from build123d import *

# Parameters (mm, degrees)
SKETCH_1_W          = 170
SKETCH_1_H          = 200
SKETCH_1_R          = 1.6
SKETCH_1_W_2        = 65
SKETCH_1_H_2        = 160
EXTRUDE_1_DEPTH     = 5
SKETCH_5_W          = 5
SKETCH_5_H          = 200
EXTRUDE_2_DEPTH     = 20
SKETCH_4_R          = 1.75
CUT_EXTRUDE_1_DEPTH = 30
SKETCH_6_W          = 5
SKETCH_6_H          = 200
EXTRUDE_3_DEPTH     = 20
CUT_EXTRUDE_2_DEPTH = 20


with BuildPart() as part:
    # 草图1 → 凸台-拉伸1 (new body)
    with BuildSketch(Plane.XY):
        with Locations((0.050009972, 0.429149843)):
            Rectangle(SKETCH_1_W, SKETCH_1_H)
        with Locations((-74.949990028, 60.429149843)):
            Circle(SKETCH_1_R, mode=Mode.SUBTRACT)
        with Locations((-74.949990028, -59.570850157)):
            Circle(SKETCH_1_R, mode=Mode.SUBTRACT)
        with Locations((75.050009972, -59.570850157)):
            Circle(SKETCH_1_R, mode=Mode.SUBTRACT)
        with Locations((75.050009972, 60.429149843)):
            Circle(SKETCH_1_R, mode=Mode.SUBTRACT)
        with Locations((75.050009972, 30.429149843)):
            Circle(SKETCH_1_R, mode=Mode.SUBTRACT)
        with Locations((-74.949990028, 30.429149843)):
            Circle(SKETCH_1_R, mode=Mode.SUBTRACT)
        with Locations((45.050009972, -59.570850157)):
            Circle(SKETCH_1_R, mode=Mode.SUBTRACT)
        with Locations((-74.949990028, 0.429149843)):
            Circle(SKETCH_1_R, mode=Mode.SUBTRACT)
        with Locations((75.050009972, 0.429149843)):
            Circle(SKETCH_1_R, mode=Mode.SUBTRACT)
        with Locations((-74.949990028, -29.570850157)):
            Circle(SKETCH_1_R, mode=Mode.SUBTRACT)
        with Locations((75.050009972, -29.570850157)):
            Circle(SKETCH_1_R, mode=Mode.SUBTRACT)
        with Locations((-44.949990028, -59.570850157)):
            Circle(SKETCH_1_R, mode=Mode.SUBTRACT)
        with Locations((45.050009972, 60.429149843)):
            Circle(SKETCH_1_R, mode=Mode.SUBTRACT)
        with Locations((-44.949990028, 60.429149843)):
            Circle(SKETCH_1_R, mode=Mode.SUBTRACT)
        with Locations((-7.449990028, 0.429149843)):
            Rectangle(SKETCH_1_W_2, SKETCH_1_H_2, mode=Mode.SUBTRACT)
    extrude(amount=EXTRUDE_1_DEPTH)

    # 草图5 → 凸台-拉伸2 (add)
    with BuildSketch(Plane.ZY.offset(84.949990028)):
        with Locations((2.5, 0.429149843)):
            Rectangle(SKETCH_5_W, SKETCH_5_H)
    extrude(amount=EXTRUDE_2_DEPTH)

    # 草图4 → 切除-拉伸1 (cut)
    with BuildSketch(Plane.XY.offset(5)):
        with BuildLine():
            Line((-99.949990028, 42.219149843), (-99.949990028, 43.969149843))
            Line((-99.949990028, 43.969149843), (-98.199990028, 43.969149843))
            ThreePointArc((-98.199990028, 43.969149843), (-101.187426895, 45.206586711), (-99.949990028, 42.219149843))
        make_face()
        with BuildLine():
            Line((-98.199990028, 43.969149843), (-99.949990028, 43.969149843))
            Line((-99.949990028, 43.969149843), (-99.949990028, 42.219149843))
            ThreePointArc((-99.949990028, 42.219149843), (-98.712553161, 42.731712976), (-98.199990028, 43.969149843))
        make_face()
        with BuildLine():
            Line((-99.949990028, 42.219149843), (-99.949990028, 43.969149843))
            Line((-99.949990028, 43.969149843), (-98.199990028, 43.969149843))
            ThreePointArc((-98.199990028, 43.969149843), (-101.187426895, 45.206586711), (-99.949990028, 42.219149843))
        make_face()
        with BuildLine():
            Line((-98.199990028, 43.969149843), (-99.949990028, 43.969149843))
            Line((-99.949990028, 43.969149843), (-99.949990028, 42.219149843))
            ThreePointArc((-99.949990028, 42.219149843), (-98.712553161, 42.731712976), (-98.199990028, 43.969149843))
        make_face()
        with BuildLine():
            ThreePointArc((-98.199990028, -43.110850157), (-98.712553161, -41.873413289), (-99.949990028, -41.360850157))
            Line((-99.949990028, -41.360850157), (-99.949990028, -43.110850157))
            Line((-99.949990028, -43.110850157), (-98.199990028, -43.110850157))
        make_face()
        with BuildLine():
            Line((-99.949990028, -43.110850157), (-99.949990028, -41.360850157))
            ThreePointArc((-99.949990028, -41.360850157), (-101.187426895, -44.348287024), (-98.199990028, -43.110850157))
            Line((-98.199990028, -43.110850157), (-99.949990028, -43.110850157))
        make_face()
        with BuildLine():
            ThreePointArc((-98.199990028, -43.110850157), (-98.712553161, -41.873413289), (-99.949990028, -41.360850157))
            Line((-99.949990028, -41.360850157), (-99.949990028, -43.110850157))
            Line((-99.949990028, -43.110850157), (-98.199990028, -43.110850157))
        make_face()
        with BuildLine():
            Line((-99.949990028, -43.110850157), (-99.949990028, -41.360850157))
            ThreePointArc((-99.949990028, -41.360850157), (-101.187426895, -44.348287024), (-98.199990028, -43.110850157))
            Line((-98.199990028, -43.110850157), (-99.949990028, -43.110850157))
        make_face()
        with BuildLine():
            ThreePointArc((-48.989990028, -43.110850157), (-49.502553161, -41.873413289), (-50.739990028, -41.360850157))
            Line((-50.739990028, -41.360850157), (-50.739990028, -43.110850157))
            Line((-50.739990028, -43.110850157), (-52.489990028, -43.110850157))
            ThreePointArc((-52.489990028, -43.110850157), (-50.739990028, -44.860850157), (-48.989990028, -43.110850157))
        make_face()
        with BuildLine():
            Line((-50.739990028, -43.110850157), (-50.739990028, -41.360850157))
            ThreePointArc((-50.739990028, -41.360850157), (-51.977426895, -41.873413289), (-52.489990028, -43.110850157))
            Line((-52.489990028, -43.110850157), (-50.739990028, -43.110850157))
        make_face()
        with BuildLine():
            ThreePointArc((-48.989990028, -43.110850157), (-49.502553161, -41.873413289), (-50.739990028, -41.360850157))
            Line((-50.739990028, -41.360850157), (-50.739990028, -43.110850157))
            Line((-50.739990028, -43.110850157), (-52.489990028, -43.110850157))
            ThreePointArc((-52.489990028, -43.110850157), (-50.739990028, -44.860850157), (-48.989990028, -43.110850157))
        make_face()
        with BuildLine():
            Line((-50.739990028, -43.110850157), (-50.739990028, -41.360850157))
            ThreePointArc((-50.739990028, -41.360850157), (-51.977426895, -41.873413289), (-52.489990028, -43.110850157))
            Line((-52.489990028, -43.110850157), (-50.739990028, -43.110850157))
        make_face()
        with Locations((-50.739990028, 43.969149843)):
            Circle(SKETCH_4_R)
    extrude(amount=-CUT_EXTRUDE_1_DEPTH, mode=Mode.SUBTRACT)

    # 草图6 → 凸台-拉伸3 (add)
    with BuildSketch(Plane(origin=(85.050009972, 0, 0), x_dir=(0, 0, -1), z_dir=(1, 0, 0))):
        with Locations((-2.5, 0.429149843)):
            Rectangle(SKETCH_6_W, SKETCH_6_H)
    extrude(amount=EXTRUDE_3_DEPTH)

    # 草图7 → 切除-拉伸2 (cut)
    with BuildSketch(Plane.XY.offset(5)):
        with BuildLine():
            Line((43.000009972, 32.029149843), (43.000009972, 33.779149843))
            Line((43.000009972, 33.779149843), (44.750009972, 33.779149843))
            ThreePointArc((44.750009972, 33.779149843), (41.762573105, 35.016586711), (43.000009972, 32.029149843))
        make_face()
        with BuildLine():
            Line((44.750009972, 33.779149843), (43.000009972, 33.779149843))
            Line((43.000009972, 33.779149843), (43.000009972, 32.029149843))
            ThreePointArc((43.000009972, 32.029149843), (44.237446839, 32.541712976), (44.750009972, 33.779149843))
        make_face()
        with BuildLine():
            Line((43.000009972, 32.029149843), (43.000009972, 33.779149843))
            Line((43.000009972, 33.779149843), (44.750009972, 33.779149843))
            ThreePointArc((44.750009972, 33.779149843), (41.762573105, 35.016586711), (43.000009972, 32.029149843))
        make_face()
        with BuildLine():
            Line((44.750009972, 33.779149843), (43.000009972, 33.779149843))
            Line((43.000009972, 33.779149843), (43.000009972, 32.029149843))
            ThreePointArc((43.000009972, 32.029149843), (44.237446839, 32.541712976), (44.750009972, 33.779149843))
        make_face()
        with BuildLine():
            ThreePointArc((44.750009972, -32.920850157), (44.237446839, -31.683413289), (43.000009972, -31.170850157))
            Line((43.000009972, -31.170850157), (43.000009972, -32.920850157))
            Line((43.000009972, -32.920850157), (44.750009972, -32.920850157))
        make_face()
        with BuildLine():
            Line((43.000009972, -32.920850157), (43.000009972, -31.170850157))
            ThreePointArc((43.000009972, -31.170850157), (41.762573105, -34.158287024), (44.750009972, -32.920850157))
            Line((44.750009972, -32.920850157), (43.000009972, -32.920850157))
        make_face()
        with BuildLine():
            ThreePointArc((44.750009972, -32.920850157), (44.237446839, -31.683413289), (43.000009972, -31.170850157))
            Line((43.000009972, -31.170850157), (43.000009972, -32.920850157))
            Line((43.000009972, -32.920850157), (44.750009972, -32.920850157))
        make_face()
        with BuildLine():
            Line((43.000009972, -32.920850157), (43.000009972, -31.170850157))
            ThreePointArc((43.000009972, -31.170850157), (41.762573105, -34.158287024), (44.750009972, -32.920850157))
            Line((44.750009972, -32.920850157), (43.000009972, -32.920850157))
        make_face()
        with BuildLine():
            ThreePointArc((96.800009972, -32.920850157), (96.287446839, -31.683413289), (95.050009972, -31.170850157))
            Line((95.050009972, -31.170850157), (95.050009972, -32.920850157))
            Line((95.050009972, -32.920850157), (93.300009972, -32.920850157))
            ThreePointArc((93.300009972, -32.920850157), (95.050009972, -34.670850157), (96.800009972, -32.920850157))
        make_face()
        with BuildLine():
            Line((95.050009972, -32.920850157), (95.050009972, -31.170850157))
            ThreePointArc((95.050009972, -31.170850157), (93.812573105, -31.683413289), (93.300009972, -32.920850157))
            Line((93.300009972, -32.920850157), (95.050009972, -32.920850157))
        make_face()
        with BuildLine():
            ThreePointArc((96.800009972, -32.920850157), (96.287446839, -31.683413289), (95.050009972, -31.170850157))
            Line((95.050009972, -31.170850157), (95.050009972, -32.920850157))
            Line((95.050009972, -32.920850157), (93.300009972, -32.920850157))
            ThreePointArc((93.300009972, -32.920850157), (95.050009972, -34.670850157), (96.800009972, -32.920850157))
        make_face()
        with BuildLine():
            Line((95.050009972, -32.920850157), (95.050009972, -31.170850157))
            ThreePointArc((95.050009972, -31.170850157), (93.812573105, -31.683413289), (93.300009972, -32.920850157))
            Line((93.300009972, -32.920850157), (95.050009972, -32.920850157))
        make_face()
        with BuildLine():
            ThreePointArc((96.800009972, 33.779149843), (95.050009972, 35.529149843), (93.300009972, 33.779149843))
            Line((93.300009972, 33.779149843), (95.050009972, 33.779149843))
            Line((95.050009972, 33.779149843), (95.050009972, 32.029149843))
            ThreePointArc((95.050009972, 32.029149843), (96.287446839, 32.541712976), (96.800009972, 33.779149843))
        make_face()
        with BuildLine():
            Line((95.050009972, 33.779149843), (93.300009972, 33.779149843))
            ThreePointArc((93.300009972, 33.779149843), (93.812573105, 32.541712976), (95.050009972, 32.029149843))
            Line((95.050009972, 32.029149843), (95.050009972, 33.779149843))
        make_face()
        with BuildLine():
            ThreePointArc((96.800009972, 33.779149843), (95.050009972, 35.529149843), (93.300009972, 33.779149843))
            Line((93.300009972, 33.779149843), (95.050009972, 33.779149843))
            Line((95.050009972, 33.779149843), (95.050009972, 32.029149843))
            ThreePointArc((95.050009972, 32.029149843), (96.287446839, 32.541712976), (96.800009972, 33.779149843))
        make_face()
        with BuildLine():
            Line((95.050009972, 33.779149843), (93.300009972, 33.779149843))
            ThreePointArc((93.300009972, 33.779149843), (93.812573105, 32.541712976), (95.050009972, 32.029149843))
            Line((95.050009972, 32.029149843), (95.050009972, 33.779149843))
        make_face()
    extrude(amount=-CUT_EXTRUDE_2_DEPTH, mode=Mode.SUBTRACT)


solid = part.part
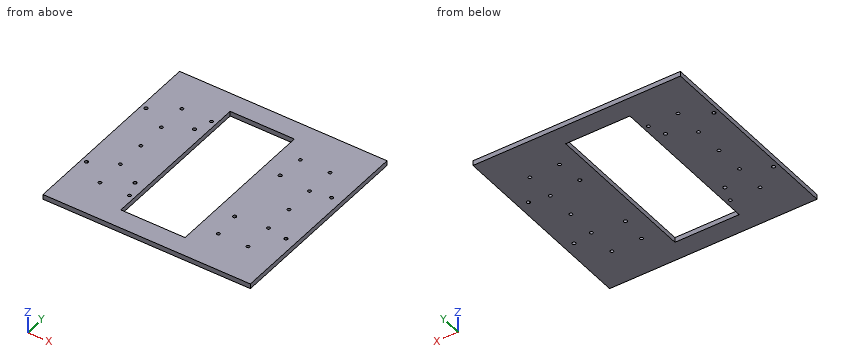
Verification items for the finished model (mm, model axes). Coordinates: 2 decimals unless noted, no trailing zeros. Order: outer loops, then holes, each group sorted by start corner. A loop starts at its lowest first (then second) coordinate and runs counter-clockwise, first axis right, second up. Notation, with made-up numbers: (33, 9.25) -> (53, 9.25) arc R24 ccw to (53, 28.25) -> close; hole circle Ø7 at (66, 68.5). An arc over 180 degrees is marked (long way). Use CSV: the item, a comma, the result in double quotes. Start each with the question number.
Q1. Depth check by flat-ended pin: P1, Ø3, axis at x = -74.95, y = -59.57, coming from the +Z side. Enter the tip coordinate at first touch or a pass-through.
Q2. Thickness scan on line 1 along X through (y, z) = (-25, 4.4); line 2 along Y through (x, z) = (15, 0.85); line 3 along X through (y, z) = (30.5, 4.7). Record the ranges inside material, lowest first.
Q3. Section check B-B, the plane x = 10. Record the cut outline in (y, z), and give its area (3 significant figures).
Q4. Section check A-A, the plane y = -54. Record the cut outline in (x, z), and give its area (3 significant figures).
Q5. Section check C-C, the plane z = 2.35. Give the number of separate pieces and of enclosed holes in the cut face, and give its area (3 significant figures).
Returned:
1,P1,"passes through"
2,line 1,"x = -104.95 to -39.95, 25.05 to 105.05"
2,line 2,"y = -99.57 to -79.57, 80.43 to 100.43"
2,line 3,"x = -104.95 to -76.55, -73.35 to -39.95, 25.05 to 73.45, 76.65 to 105.05"
3,outline,"(-99.57, 0) -> (-79.57, 0) -> (-79.57, 5) -> (-99.57, 5) -> close; (80.43, 0) -> (100.43, 0) -> (100.43, 5) -> (80.43, 5) -> close"
3,area,"200 mm^2"
4,outline,"(-104.95, 0) -> (-39.95, 0) -> (-39.95, 5) -> (-104.95, 5) -> close; (25.05, 0) -> (105.05, 0) -> (105.05, 5) -> (25.05, 5) -> close"
4,area,"725 mm^2"
5,separate pieces,"1"
5,enclosed holes,"23"
5,area,"31,400 mm^2"
